Design review of the part shown in the three views and the two pictorial views. Dimensions are in mm from the part's minimum x, y and z. Give positions to 0.01 mm unless a question says otherwise; leave off trailing zeros. Write each loop counter-clockwise with the first axis right and the second up, starting at its lowest first coordinate (ties: lowest second). Pieces come first, ordered by that corner, then holes.
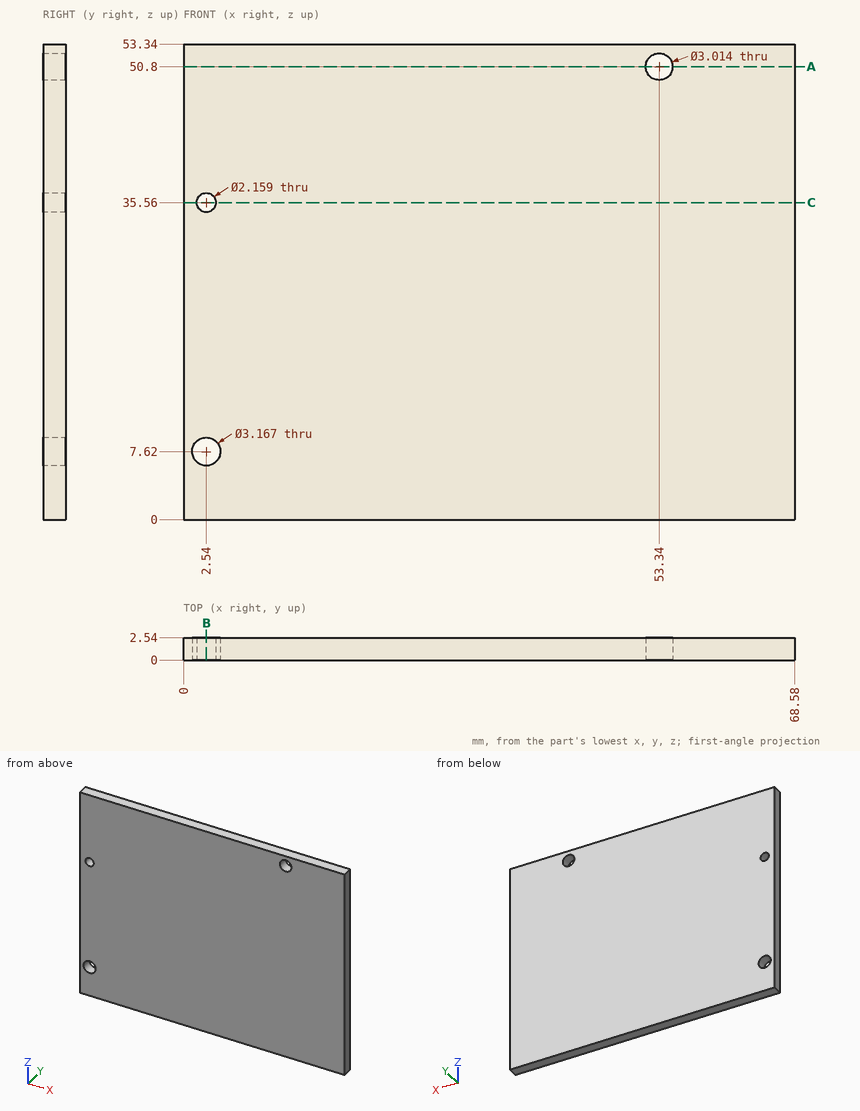
(1) Consider section C-C, the plane z = 35.56. Give the boundary of the cut face in (x, y), then the cut area to 3 significant figures.
Resolved:
outline: (0, 0) - (1.46, 0) - (1.46, 2.54) - (0, 2.54) - close; (3.62, 0) - (68.58, 0) - (68.58, 2.54) - (3.62, 2.54) - close
area: 169 mm2
(2) Consider section B-B, the plane x = 2.54. Give the boundary of the cut face in (y, z).
Resolved:
outline: (0, 0) - (2.54, 0) - (2.54, 6.04) - (0, 6.04) - close; (0, 9.2) - (2.54, 9.2) - (2.54, 34.48) - (0, 34.48) - close; (0, 36.64) - (2.54, 36.64) - (2.54, 53.34) - (0, 53.34) - close
(3) Consider section A-A, the plane z = 50.8. Give the boundary of the cut face in (x, y), then the cut area to 3 significant figures.
Resolved:
outline: (0, 0) - (51.83, 0) - (51.83, 2.54) - (0, 2.54) - close; (54.85, 0) - (68.58, 0) - (68.58, 2.54) - (54.85, 2.54) - close
area: 167 mm2
(4) To check wall thickness, follow L1, parallel to X at y = 0.75, z = 7.62; L2, parallel to X at y = 2, z = 35.56. State the ranges of each line that lie inside material, in increasing order.
Resolved:
L1: x = 0 to 0.96, 4.12 to 68.58
L2: x = 0 to 1.46, 3.62 to 68.58
(5) Clearance check with flat-ended pins moving along their axes: P1, Ø1.5, axis at x = 32, z = 6, coming from the -Y side; P2, Ø2.5, axis at x = 2.54, z = 7.62, coming from the -Y side. State where each tip first meets the part, or that it passes through.
Resolved:
P1: stops at y = 0
P2: passes through
